The listing builds one solid part. Answer for the finished solid, in the listing's coordinates (mm). A direction names the side the tool comes from. Give positions to 0.01 mm unless a question says otherwise; leave off trailing zeros. Order: outer loops, then holes, each group sorted by start corner. A loop starts at its lowest first (then second) coordinate and runs counter-clockwise, first axis right, second up. Notation, with made-up numbers: (3.5, -2.75) - (39.5, -2.75) arc R19 ccw to (39.5, 29.25) - close; hole circle Ø8 at (14, 7.25). An arc over 180 degrees is marked (long way). Answer as a JSON object with one key per item and string values. Group by question number.
Q1. Consider line 1 (Z direction, x = -12.55, y = 0); line 2 (Y direction, x = 3, z = 7); line 3 (Z direction, x = 37.5, y = -4.5). Determine where each line is inside the solid, lowest interval first.
Q2. A cutting plane is placed at D-D, the plane y = 2.75. Give the vertices of the cut face in (x, z).
Q3. A cutting plane is placed at C-C, the plane x = -1. Give the vertices of the cut face in (y, z).
Q4. For faces 4 (the face through (-18.4, 2.4, 3)), 5 (the face through (38, -2, 2)), 6 (the face through (14.161, 0, 2)), 7 (the face through (32, 0, 3)), determine the directions among +Z, -Z, +X, -X, +Y, -Y from which every point of the face is accessible in a straight line to the end or side of a thin tool.
Q5. Given pin 1 (5 mm diameter, centred on x = 13.5, z = 16.5, fed in from -Y) (1 decimal); pin 2 (2.5 mm diameter, centred on y = 4.5, z = 7, fed in from +X); pin 3 (5.5 mm diameter, centred on y = -2, z = 14.5, fed in from -X); pin 4 (4.5 mm diameter, centred on x = 18, y = -1.5, fed in from +Z), each flat-ended and moving along its own axis, determine where each tip first touches the part or whether it passes through.
Q6. The mould has two halves that part along Y. Classify faces 1 (the face through (-20, -2, 2)), 2 (the face through (-19.867, -8.479, 1.521)), 3 (the face through (24.72, -0.14, 14.96)): released by +Y, released by -Y, zero draft, split by the parting line, or undercut.
Q7. A cutting plane is placed at A-A, the plane y = 0. Give the vertices of the cut face in (x, z), and give its area (3 significant figures).
Q8. A cutting plane is placed at B-B, the plane z = 5.5. Give the vertices of the cut face in (x, y), and give its area (3 significant figures).
from build123d import *

# Parameters (mm, degrees)
F1_DEPTH  = 10
F3_W      = 4
F3_H      = 4
F4_DEPTH  = 3
F5_DEPTH  = 3
F7_DEPTH  = 3
F8_DEPTH  = 3
F9_W      = 16
F9_H      = 4
F10_DEPTH = 6
F11_DEPTH = 3
F12_R     = 3.5
F13_DEPTH = 3


with BuildPart() as f1:
    # F0 (on Front) → F1 (new body, symmetric)
    with BuildSketch(Plane.XZ):
        Polygon((-17.8393546607, 3), (-17.8393546607, 0), (-7.8393546607, 0), (-7.8393546607, 3), (14.1606453393, 3), (14.1606453393, 0), (36.1606453393, 0), (36.1606453393, 3), (29.1606453393, 3), (29.1606453393, 11), (20.1606453393, 19.0285857916), (16.1606453393, 19.0285857916), (16.1606453393, 8.0285857916), (-11.8393546607, 8.0285857916), (-11.8393546607, 10.0285857916), (-14.8393546607, 10.0285857916), (-14.8393546607, 3), align=None)
    extrude(amount=F1_DEPTH, both=True)

    # F3 (on face) → F4 (join)
    with BuildSketch(Plane.XY.offset(3)):
        Polygon((40.1606453393, 7), (36.1606453393, 10), (36.1606453393, 2), (40.1606453393, 2), align=None)
        Polygon((40.1606453393, 10), (36.1606453393, 10), (40.1606453393, 7), align=None)
        with Locations((38.1606453393, 0)):
            Rectangle(F3_W, F3_H)
        with BuildLine():
            Line((36.1606453393, -2), (36.1606453393, 2))
            Line((36.1606453393, 2), (35.1606453393, 2))
            ThreePointArc((35.1606453393, 2), (33.1606453393, 0), (35.1606453393, -2))
            Line((35.1606453393, -2), (36.1606453393, -2))
        make_face()
        Polygon((40.1606453393, -2), (36.1606453393, -2), (36.1606453393, -10), (40.1606453393, -7), align=None)
        Polygon((40.1606453393, -7), (36.1606453393, -10), (40.1606453393, -10), align=None)
    extrude(amount=-F4_DEPTH)

    # F3 (on face) → F5 (cut)
    with BuildSketch(Plane.XY.offset(3)):
        with Locations((38.1606453393, 0)):
            Rectangle(F3_W, F3_H)
        with BuildLine():
            Line((36.1606453393, -2), (36.1606453393, 2))
            Line((36.1606453393, 2), (35.1606453393, 2))
            ThreePointArc((35.1606453393, 2), (33.1606453393, 0), (35.1606453393, -2))
            Line((35.1606453393, -2), (36.1606453393, -2))
        make_face()
        Polygon((40.1606453393, -7), (36.1606453393, -10), (40.1606453393, -10), align=None)
        Polygon((40.1606453393, 10), (36.1606453393, 10), (40.1606453393, 7), align=None)
    extrude(amount=-F5_DEPTH, mode=Mode.SUBTRACT)

    # F6 (on face) → F7 (join)
    with BuildSketch(Plane.XY.offset(3)):
        Polygon((-17.8393546607, 2), (-17.8393546607, 10), (-21.8393546607, 7), (-21.8393546607, 2), align=None)
        Polygon((-17.8393546607, -10), (-17.8393546607, -2), (-21.8393546607, -2), (-21.8393546607, -7), align=None)
    extrude(amount=-F7_DEPTH)

    # F6 (on face) → F8 (cut)
    with BuildSketch(Plane.XY.offset(3)):
        with BuildLine():
            ThreePointArc((-17.8393546607, -2), (-15.8393546607, 0), (-17.8393546607, 2))
            Line((-17.8393546607, 2), (-17.8393546607, -2))
        make_face()
    extrude(amount=-F8_DEPTH, mode=Mode.SUBTRACT)

    # F9 (on face) → F10 (cut)
    with BuildSketch(Plane(origin=(0, 0, 3), x_dir=(1, 0, 0), z_dir=(0, 0, -1))):
        with Locations((3.1606453393, 0)):
            Rectangle(F9_W, F9_H)
        with BuildLine():
            Line((-4.8393546607, -2), (-4.8393546607, 2))
            ThreePointArc((-4.8393546607, 2), (-6.8393546607, 0), (-4.8393546607, -2))
        make_face()
        with BuildLine():
            ThreePointArc((11.1606453393, -2), (13.1606453393, 0), (11.1606453393, 2))
            Line((11.1606453393, 2), (11.1606453393, -2))
        make_face()
    extrude(amount=-F10_DEPTH, mode=Mode.SUBTRACT)

    # F2 (on face) → F11 (join)
    with BuildSketch(Plane.YZ.offset(-11.8393546607)):
        with BuildLine():
            Line((-10, 10.0285857916), (10, 10.0285857916))
            ThreePointArc((10, 10.0285857916), (0, 20.0285857916), (-10, 10.0285857916))
        make_face()
    extrude(amount=-F11_DEPTH)

    # F12 (on face) → F13 (cut)
    with BuildSketch(Plane.YZ.offset(-11.8393546607)):
        with Locations((0, 13.5285857916)):
            Circle(F12_R)
    extrude(amount=-F13_DEPTH, mode=Mode.SUBTRACT)


solid = f1.part
Reply:
{
 "1": {"line 1": "z = 0 to 10.03, 17.03 to 20.03", "line 2": "y = -10 to -2, 2 to 10", "line 3": "z = 0 to 3"},
 "2": {"outline": "(-21.84, 0) - (-7.84, 0) - (-7.84, 3) - (14.16, 3) - (14.16, 0) - (40.16, 0) - (40.16, 3) - (29.16, 3) - (29.16, 11) - (20.16, 19.03) - (16.16, 19.03) - (16.16, 8.03) - (-11.84, 8.03) - (-11.84, 11.36) - (-14.84, 11.36) - (-14.84, 3) - (-21.84, 3) - close; (-14.84, 15.69) - (-11.84, 15.69) - (-11.84, 19.64) - (-14.84, 19.64) - close"},
 "3": {"outline": "(-10, 3) - (-2, 3) - (-2, 8.03) - (-10, 8.03) - close; (2, 3) - (10, 3) - (10, 8.03) - (2, 8.03) - close"},
 "4": {"face 4": "+Z, -X, +Y, -Y", "face 5": "+Z, -Z, +X", "face 6": "-Z, +Y, -Y", "face 7": "+Z, +X, +Y, -Y"},
 "5": {"pin 1": "passes through", "pin 2": "stops at x = 29.16", "pin 3": "stops at x = -14.84", "pin 4": "stops at z = 19.03"},
 "6": {"face 1": "undercut", "face 2": "released by -Y", "face 3": "zero draft"},
 "7": {"outline": "(-15.84, 0) - (-7.84, 0) - (-7.84, 3) - (-6.84, 3) - (-6.84, 8.03) - (-11.84, 8.03) - (-11.84, 10.03) - (-14.84, 10.03) - (-14.84, 3) - (-15.84, 3) - close; (-14.84, 17.03) - (-11.84, 17.03) - (-11.84, 20.03) - (-14.84, 20.03) - close; (13.16, 3) - (14.16, 3) - (14.16, 0) - (33.16, 0) - (33.16, 3) - (29.16, 3) - (29.16, 11) - (20.16, 19.03) - (16.16, 19.03) - (16.16, 8.03) - (13.16, 8.03) - close", "area": "324 mm^2"},
 "8": {"outline": "(-14.84, -10) - (29.16, -10) - (29.16, 10) - (-14.84, 10) - close; hole (-4.84, -2) - (11.16, -2) arc R2 ccw to (11.16, 2) - (-4.84, 2) arc R2 ccw to start", "area": "803 mm^2"}
}
